Autodesk Fusion 360 part; units mm, degrees
sketch "Sketch1" plane through (0, 0, 0) normal (0, 1, 0) x (1, 0, 0)
  circle A0 centre (0, 0) radius 51
  circle A1 centre (0, 0) radius 48.75
  circle A2 centre (0, 0) radius 38
  dimension "d1" = 102
  dimension "d2" = 97.5
  dimension "d3" = 76
extrude "Extrude1" add sketch "Sketch1" along normal blind 2 contours A0 | A1 | A2
extrude "Extrude2" add sketch "Sketch1" against normal blind 15 contours A1
extrude "Extrude3" add sketch "Sketch1" against normal blind 58 contours A0
extrude "Extrude4" cut 1 faces at (44.8437, -15, 4.3098) along direction (0, 1, 0) up to surface (15 mm away)
extrude "Extrude5" cut sketch "Sketch1" along normal blind 20 contours A1 | A2
Geometry check sheet. Reference: the model listing, model coordinates, mm. Give positions to 0.01 mm unless a question says otherwise; leave off trailing zeros. Order: outer loops, then holes, each group sorted by start corner. A loop starts at its lowest first (then second) coordinate and runs counter-clockwise, first axis right, second up.
1. Section check C-C, the plane y = -44. Enter the section's corners in (x, z).
2. Thickness scan on L1, parallel to X at y = -19, z = 0; L2, parallel to X at y = -16.5, z = -18. Record the ranges inside material, lowest first.
3. Release check for a two-part mould opening along X. For faces 1 (the face through (-38.69, -27.58, 29.66)), 2 (the face through (41.3, 2, 26.2)), 3 (the face through (-11.056, -27.58, 49.787)) record: pulls with the +X half, pulls with the -X half, needs draft (parallel to the pull), parting line crosses it, or undercut.
4. Section check A-A, the plane z = 0. Enter the section's corners in (x, y).
5. Gauge pin test, flat ends, axial feed: pin 1 Ø1.5 at (y, z) = (-14, -5) entering from +X; pin 2 Ø8 at (y, z) = (-7, -10.5) entering from +X; pin 3 Ø8 at (y, z) = (-28, 21) entering from +X; pin 4 Ø12 at (y, z) = (-28, -6) entering from +X. Record the tip position at first contact, or that the pin passes through.
6. Section check B-B, the plane x = 0. Enter the section's corners in (y, z), and give its area (3 significant figures).
Values follow:
1. outline: circle Ø102 at (0, 0); hole circle Ø97.5 at (0, 0)
2. L1: x = -51 to -48.75, 48.75 to 51
2. L2: x = -47.72 to -45.31, 45.31 to 47.72
3. face 1: undercut
3. face 2: needs draft
3. face 3: parting line crosses it
4. outline: (-51, -58) - (-48.75, -58) - (-48.75, 2) - (-51, 2) - close; (48.75, -58) - (51, -58) - (51, 2) - (48.75, 2) - close
5. pin 1: stops at x = 50.82
5. pin 2: stops at x = 50.58
5. pin 3: stops at x = 48.08
5. pin 4: stops at x = 51
6. outline: (-58, -51) - (2, -51) - (2, -48.75) - (-58, -48.75) - close; (-58, 48.75) - (2, 48.75) - (2, 51) - (-58, 51) - close
6. area: 270 mm2
